Build history of the part. All positions in model axes, mm. Give positions to 0.01 mm unless a question says otherwise; leave off trailing zeros. Write each loop counter-clockwise with the first axis right and the second up, starting at its lowest first coordinate (ties: lowest second). Pieces come first, ordered by that corner, then holes.
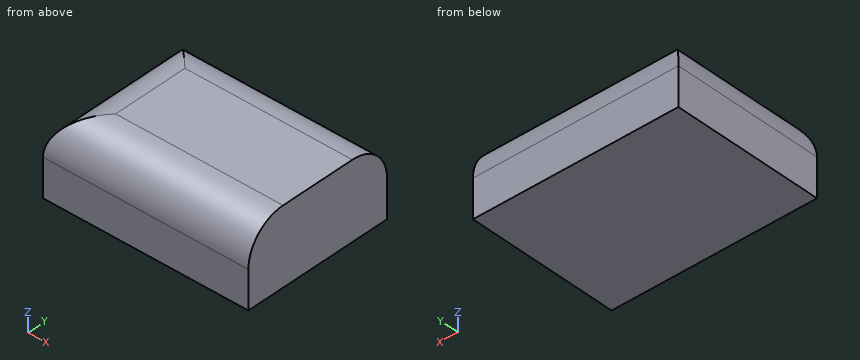
from build123d import *

# Parameters (mm, degrees)
SKETCH1_W           = 63.5
SKETCH1_H           = 127
BOSS_EXTRUDE1_DEPTH = 171.45
FILLET1_R           = 31.75


with BuildPart() as part:
    # Sketch1 → Boss-Extrude1 (new body)
    with BuildSketch(Plane(origin=(0, 0, 0), x_dir=(0, 0, -1), z_dir=(1, 0, 0))):
        with Locations((-5.766791516, 21.358919545)):
            Rectangle(SKETCH1_W, SKETCH1_H)
    extrude(amount=BOSS_EXTRUDE1_DEPTH)

    # Fillet1
    fillet1_edges = [part.edges().sort_by_distance(p)[0] for p in [
        (0, 21.358919545, 37.516791516),
        (85.725, 84.858919545, 37.516791516),
        (85.725, -42.141080455, 37.516791516),
    ]]
    fillet(fillet1_edges, radius=FILLET1_R)


solid = part.part
(1) Saw through at C-C, the plane y = -31. List the corners of the cut face in (x, z).
(2) Drop flat-ended pins along their axis: pin 1 (1.5 mm diameter, centred on x = 135, z = 23, fed in from +Y) (3 decimals); pin 2 (4 mm diameter, centred on x = 105, z = 30.5, fed in from -Y); pin 3 (8 mm diameter, centred on x = 100, z = 25.5, fed in from +Y). Give the stop position or say it passes through.
(3) Saw through at B-B, the plane x = 140. List the corners of the cut face in (y, z).
(4) Saw through at A-A, the plane y = 11. List the corners of the cut face in (x, z), plus the area to 3 significant figures.
(5) Probe line 1 (Y direction, x = 52, z = 27); line 2 (X direction, y = 79, z = 11.5); line 3 (X direction, y = 63, z = 21.5). List the from-to ranges inside material, lowest first.
Computed values:
1. outline: (0, -25.98) - (171.45, -25.98) - (171.45, 29.92) - (11.14, 29.92) arc R31.75 ccw to (0, 5.77) - close
2. pin 1: stops at y = 80.245
2. pin 2: stops at y = -32.56
2. pin 3: stops at y = 80.69
3. outline: (-42.14, -25.98) - (84.86, -25.98) - (84.86, 5.77) arc R31.75 ccw to (53.11, 37.52) - (-10.39, 37.52) arc R31.75 ccw to (-42.14, 5.77) - close
4. outline: (0, -25.98) - (171.45, -25.98) - (171.45, 37.52) - (31.75, 37.52) arc R31.75 ccw to (0, 5.77) - close
4. area: 10,700 mm2
5. line 1: y = -34 to 76.71
5. line 2: x = 0.52 to 171.45
5. line 3: x = 4.17 to 171.45
